Source: CAD feature listing. Evaluate the final solid. Frame: model axes, mm. Face numbers are marked on the shaded views. A direction names the side the tool comes from. Give positions to 0.01 mm unless a question says otherwise; leave off trailing zeros. Order: outer loops, then holes, each group sorted by start corner. A loop starts at its lowest first (then second) coordinate and runs counter-clockwise, first axis right, second up. Notation, with made-up numbers: (56, -13.5) -> (115, -13.5) arc R31 cw to (115, 14.5) -> close; hole circle Ø2 at (46.25, 54.5). An arc over 180 degrees is marked (long way). Use CSV: the item, a comma, the result in double quotes.
```python
from build123d import *

# Parameters (mm, degrees)
SKETCH028_W     = 77
SKETCH028_H     = 50
SKETCH028_R     = 2.5
SKETCH028_W_2   = 28
SKETCH028_H_2   = 28
PAD018_DEPTH    = 1
SKETCH029_R     = 1.4
PAD019_DEPTH    = 5
SKETCH030_W     = 73
SKETCH030_H     = 46
SKETCH030_W_2   = 71.2
SKETCH030_H_2   = 44.2
PAD020_DEPTH    = 10
SKETCH031_W     = 10
SKETCH031_H     = 3
POCKET004_DEPTH = 5
SKETCH032_W     = 10
SKETCH032_H     = 30
PAD021_DEPTH    = 2


with BuildPart() as part:
    # Sketch028 → Pad018 (new body)
    with BuildSketch(Plane.XY):
        with Locations((38.5, 25)):
            Rectangle(SKETCH028_W, SKETCH028_H)
        with Locations((11, 32.5)):
            Circle(SKETCH028_R, mode=Mode.SUBTRACT)
        with Locations((11, 25)):
            Circle(SKETCH028_R, mode=Mode.SUBTRACT)
        with Locations((11, 17.5)):
            Circle(SKETCH028_R, mode=Mode.SUBTRACT)
        with Locations((45, 25)):
            Rectangle(SKETCH028_W_2, SKETCH028_H_2, mode=Mode.SUBTRACT)
    extrude(amount=PAD018_DEPTH)

    # Sketch029 → Pad019 (join)
    with BuildSketch(Plane.XY.offset(1)):
        with Locations((26.5, 39)):
            Circle(SKETCH029_R)
        with Locations((69.5, 39)):
            Circle(SKETCH029_R)
        with Locations((69.5, 11)):
            Circle(SKETCH029_R)
        with Locations((26.5, 11)):
            Circle(SKETCH029_R)
    extrude(amount=PAD019_DEPTH)

    # Sketch030 → Pad020 (join)
    with BuildSketch(Plane.XY.offset(1)):
        with Locations((38.5, 25)):
            Rectangle(SKETCH030_W, SKETCH030_H)
        with Locations((38.5, 25)):
            Rectangle(SKETCH030_W_2, SKETCH030_H_2, mode=Mode.SUBTRACT)
    extrude(amount=PAD020_DEPTH)

    # Sketch031 (on Face16 of Pad020) → Pocket004 (cut)
    with BuildSketch(Plane.YZ.offset(75)):
        with Locations((24.5, 9.5)):
            Rectangle(SKETCH031_W, SKETCH031_H)
    extrude(amount=-POCKET004_DEPTH, mode=Mode.SUBTRACT)

    # Sketch032 (on Face18 of Pocket004) → Pad021 (join)
    with BuildSketch(Plane.XY.offset(1)):
        with Locations((10.5, 25)):
            Rectangle(SKETCH032_W, SKETCH032_H)
        with BuildLine():
            ThreePointArc((14.007906, 33.25), (7.9, 32.5), (14.007906, 31.75))
            Line((15.007906, 31.75), (14.007906, 31.75))
            Line((15.007906, 33.25), (15.007906, 31.75))
            Line((14.007906, 33.25), (15.007906, 33.25))
        make_face(mode=Mode.SUBTRACT)
        with BuildLine():
            ThreePointArc((14.007906, 25.75), (7.9, 25), (14.007906, 24.25))
            Line((15.007906, 24.25), (14.007906, 24.25))
            Line((15.007906, 25.75), (15.007906, 24.25))
            Line((14.007906, 25.75), (15.007906, 25.75))
        make_face(mode=Mode.SUBTRACT)
        with BuildLine():
            ThreePointArc((14.007906, 18.25), (7.9, 17.5), (14.007906, 16.75))
            Line((15.007906, 16.75), (14.007906, 16.75))
            Line((15.007906, 18.25), (15.007906, 16.75))
            Line((14.007906, 18.25), (15.007906, 18.25))
        make_face(mode=Mode.SUBTRACT)
    extrude(amount=PAD021_DEPTH)


solid = part.part
```
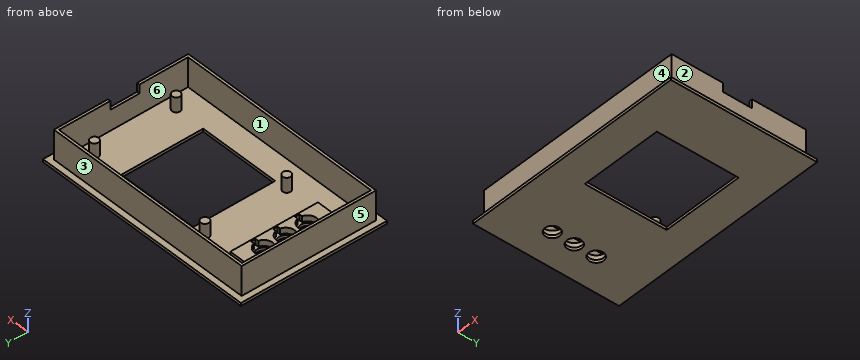
1. Section query C-C on x = 51.5. Return loops of the section in (y, z).
Answer below:
outline,"(0, 0) -> (11, 0) -> (11, 1) -> (2.9, 1) -> (2.9, 11) -> (2, 11) -> (2, 1) -> (0, 1) -> close; (39, 0) -> (50, 0) -> (50, 1) -> (48, 1) -> (48, 11) -> (47.1, 11) -> (47.1, 1) -> (39, 1) -> close"
2. Section query B-B on y = 32.5. Return loops of the section in (x, z), plus the area to 3 significant figures.
Answer below:
outline,"(0, 0) -> (8.5, 0) -> (8.5, 1) -> (7.9, 1) -> (7.9, 3) -> (5.5, 3) -> (5.5, 1) -> (2.9, 1) -> (2.9, 11) -> (2, 11) -> (2, 1) -> (0, 1) -> close; (13.5, 0) -> (31, 0) -> (31, 1) -> (15.5, 1) -> (15.5, 3) -> (15.01, 3) -> (15.01, 1) -> (13.5, 1) -> close; (59, 0) -> (77, 0) -> (77, 1) -> (75, 1) -> (75, 11) -> (74.1, 11) -> (74.1, 1) -> (59, 1) -> close"
area,"67.8 mm²"
3. Mould query, pull axis X, two halves, no side actions, for the marked faces 4, 5 and 6. Classes: released by +X, released by -X, zero draft, split by the parting line, or undercut.
Answer below:
face 4,"zero draft"
face 5,"released by -X"
face 6,"undercut"
4. Section query A-A on z = 2. Count the separate pieces of the cut face and the enclosed holes in it, plus the area to 3 significant figures.
Answer below:
separate pieces,"6"
enclosed holes,"4"
area,"441 mm²"
5. Access query for the marked faces 1, 2 and 3. Directions: +Z, -Z, +X, -X, +Y, -Y. A direction counts if a zero-diameter tool reaches every point of the face in a straight line with its end or side. Return the directions, or none.
Answer below:
face 1,"+Z"
face 2,"+Z, +X, +Y, -Y"
face 3,"+Z, +X, -X, +Y"
6. Ray query, line 1 along X through (y, z) = (25, 2.35); line 2 along Y through (x, z) = (11, 0.75); line 3 along Y through (x, z) = (11, 1.8). Return the intervals inside material, ascending.
Answer below:
line 1,"x = 2 to 2.9, 5.5 to 7.9, 15.01 to 15.5, 74.1 to 75"
line 2,"y = 0 to 15, 20 to 22.5, 27.5 to 30, 35 to 50"
line 3,"y = 2 to 2.9, 10 to 14.4, 20.6 to 21.9, 28.1 to 29.4, 35.6 to 40, 47.1 to 48"
7. Section query D-D on y = 13.5. Return loops of the section in (x, z), plus the area to 3 significant figures.
Answer below:
outline,"(0, 0) -> (31, 0) -> (31, 1) -> (15.5, 1) -> (15.5, 3) -> (5.5, 3) -> (5.5, 1) -> (2.9, 1) -> (2.9, 11) -> (2, 11) -> (2, 1) -> (0, 1) -> close; (59, 0) -> (77, 0) -> (77, 1) -> (75, 1) -> (75, 11) -> (74.1, 11) -> (74.1, 1) -> (59, 1) -> close"
area,"87.0 mm²"
8. Pin query (flat end, axial travel): P1, Ø2, axis at x = 42.5, z = 8.5, coming from the -Y side; P2, Ø5, axis at y = 9, z = 8, coming from the +X side; P3, Ø1.2, axis at y = 32.5, z = 2.5, coming from the -X side; P4, Ø4, axis at x = 69, y = 38, coming from the -Z side. Return the tip coordinate at first contact, or that it passes through.
Answer below:
P1,"stops at y = 2"
P2,"stops at x = 75"
P3,"stops at x = 2"
P4,"stops at z = 0"
